For this review, take the finished solid that the model builds, in its own axes (mm). A direction names the side the tool comes from. Give positions to 0.01 mm unless a question says otherwise; leave off trailing zeros. Loops run counter-clockwise (first coordinate to the right, second up) from the corner with the lowest first, then second, coordinate; pieces in that order, holes last. Notation, with made-up numbers: (29, -34.75) - (39, -34.75) arc R8 cw to (39, -30.75) - close; hole circle Ø3 at (-9.75, 22.25). An arc over 180 degrees is marked (long way). Use CSV: the item, a comma, the result in double quotes. Start each with the question number.
1. Take a section at A-A on y = -35. Give the boundary of the cut face in (x, z), plus the area to 3 significant figures.
2. Take a section at D-D on y = 3.5. Give the boundary of the cut face in (x, z).
3. Mouldability with a two-part tool opening along Z and no side actions: class faces 1 (the flat face through (0, -70, -5)), 2 (the cylindrical face through (0.042, 57.196, 151.917)), 3 (the flat face through (0, -15, 65)), 4 (the cylindrical face through (0.042, 73.196, 151.917)) as pulls with the +Z half, pulls with the -Z half, needs draft (parallel to the pull), parting line crosses it, or undercut.
4. Take a section at C-C on x = 0.95. State how many separate pieces and enclosed holes the cut face has, plus the area to 3 significant figures.
5. For pin 1 (2 mm diameter, centred on x = 0, z = 82, fed in from -Y); pin 2 (12 mm diameter, centred on y = -16, z = 102.5, fed in from +X); pin 3 (1 mm diameter, centred on x = 1.5, y = -17, fed in from +Z), all flat-tipped, find the tip position at first contact; note any pin that passes through.
6. Wall thickness on line 1 (Y direction, x = 1, z = 55); line 2 (Y direction, x = -1, z = 50); line 3 (Y direction, x = 2.5, z = 152): over which ranges is each line inside the solid? List them lowest first.
7. For faces 5 (the cylindrical face through (0.04, -47.05, -6.54)), 6 (the flat face through (0.042, -63.695, 13.522)), list the 3-axis set-ups (+Z, -Z, +X, -X, +Y, -Y) from which the entire face can be reached by the end or side of a thin tool; tool diameter is ignored.
8. Take a section at B-B on y = 74. Give the boundary of the cut face in (x, z), plus the area to 3 significant figures.
```python
from build123d import *

# Parameters (mm, degrees)
SKETCH_1_R               = 6.025
EXTRUDE_1_DEPTH          = 3
SKETCH_2_R               = 3
SKETCH_2_R_2             = 2.1
CUT_EXTRUDE_1_DEPTH      = 10
SKETCH_4_R               = 2.1
CUT_EXTRUDE_3_DEPTH      = 10
CHAMFER_1_SIZE           = 10
FILLET_1_R               = 3
SKETCH_5_R               = 2.1
CUT_EXTRUDE_4_DEPTH      = 10
EXTRUDE_2_DEPTH          = 6
CUT_EXTRUDE_6_DEPTH      = 182.747077005
CUT_EXTRUDE_6_DEPTH_BACK = 182.747077005
EXTRUDE_START            = -6
SKETCH_7_R               = 2.1
EXTRUDE_3_DEPTH          = 6


with BuildPart() as part:
    # 草图1 → 凸台-拉伸1 (new, symmetric)
    with BuildSketch(Plane(origin=(0, 0, 0), x_dir=(0, 0, -1), z_dir=(1, 0, 0))):
        with BuildLine():
            Line((-60, -42.021540511), (0, -70))
            Line((0, -70), (12, -70))
            Line((12, -70), (12, 30))
            Line((12, 30), (-75.715728753, 30))
            Line((-75.715728753, 30), (-125.857864376, 80.142135624))
            ThreePointArc((-125.857864376, 80.142135624), (-154.142135624, 80.142135624), (-154.142135624, 51.857864376))
            Line((-154.142135624, 51.857864376), (-92.284271247, -10))
            Line((-92.284271247, -10), (-60, -10))
            Line((-60, -10), (-60, -42.021540511))
        make_face()
        Circle(SKETCH_1_R, mode=Mode.SUBTRACT)
    extrude(amount=EXTRUDE_1_DEPTH, both=True)

    # 草图2 → 切除-拉伸1 (cut)
    with BuildSketch(Plane(origin=(3, 0, 0), x_dir=(0, 0, -1), z_dir=(1, 0, 0))):
        with Locations((-140, 66)):
            Circle(SKETCH_2_R)
        with Locations((-140, 82)):
            Circle(SKETCH_2_R_2)
        with Locations((-126.143593539, 74)):
            Circle(SKETCH_2_R_2)
        with Locations((-126.143593539, 58)):
            Circle(SKETCH_2_R_2)
        with Locations((-140, 50)):
            Circle(SKETCH_2_R_2)
        with Locations((-153.856406461, 58)):
            Circle(SKETCH_2_R_2)
        with Locations((-153.856406461, 74)):
            Circle(SKETCH_2_R_2)
    extrude(amount=-CUT_EXTRUDE_1_DEPTH, mode=Mode.SUBTRACT)

    # 草图4 → 切除-拉伸3 (cut)
    with BuildSketch(Plane(origin=(3, 0, 0), x_dir=(0, 0, -1), z_dir=(1, 0, 0))):
        with Locations((-55, -15)):
            Circle(SKETCH_4_R)
        with Locations((-55, -35)):
            Circle(SKETCH_4_R)
        with Locations((7, -65)):
            Circle(SKETCH_4_R)
        with Locations((7, -45)):
            Circle(SKETCH_4_R)
        with Locations((-8, -60.75264914)):
            Circle(SKETCH_4_R)
        with Locations((-26.126155741, -52.300283905)):
            Circle(SKETCH_4_R)
        with Locations((-44.252311481, -43.84791867)):
            Circle(SKETCH_4_R)
    extrude(amount=-CUT_EXTRUDE_3_DEPTH, mode=Mode.SUBTRACT)

    # 倒角1
    chamfer_1_edges = [part.edges().sort_by_distance(p)[0] for p in [
        (0, -10, 60),
    ]]
    chamfer(chamfer_1_edges, length=CHAMFER_1_SIZE)

    # 圆角1
    fillet_1_edges = [part.edges().sort_by_distance(p)[0] for p in [
        (0, -20, 60),
        (0, -10, 70),
        (0, 30, -12),
        (0, -70, -12),
        (0, -70, 0),
        (0, -42.021540511, 60),
        (0, -10, 92.284271247),
        (0, 30, 75.715728753),
    ]]
    fillet(fillet_1_edges, radius=FILLET_1_R)

    # 草图5 → 切除-拉伸4 (cut)
    with BuildSketch(Plane(origin=(3, 0, 0), x_dir=(0, 0, -1), z_dir=(1, 0, 0))):
        with Locations((-110, 57.213203436)):
            Circle(SKETCH_5_R)
        with Locations((-88.786796564, 36)):
            Circle(SKETCH_5_R)
        with Locations((-109.946763354, 14.785654888)):
            Circle(SKETCH_5_R)
        with Locations((-131.214342006, 35.94434337)):
            Circle(SKETCH_5_R)
        with Locations((-58, 25)):
            Circle(SKETCH_5_R)
        with Locations((-28, 25)):
            Circle(SKETCH_5_R)
    extrude(amount=-CUT_EXTRUDE_4_DEPTH, mode=Mode.SUBTRACT)

    # 草图6 → 凸台-拉伸2 (add)
    with BuildSketch(Plane.ZY.offset(3)):
        with BuildLine():
            Line((36.127383127, -53.153524579), (26.084776747, -57.836468842))
            ThreePointArc((26.084776747, -57.836468842), (30.261373424, -57.503051447), (33.637803948, -59.983947227))
            ThreePointArc((33.637803948, -59.983947227), (46.226182617, -63.56307787), (51.576063312, -51.619199512))
            ThreePointArc((51.576063312, -51.619199512), (51.845914592, -47.438014603), (54.785991728, -44.452872497))
            Line((54.785991728, -44.452872497), (44.743385348, -49.13581676))
            ThreePointArc((44.743385348, -49.13581676), (47.139529245, -51.355820594), (48.025, -54.5))
            ThreePointArc((48.025, -54.5), (41.322464636, -60.486783012), (36.127383127, -53.153524579))
        make_face()
    extrude(amount=-EXTRUDE_2_DEPTH)

    # 草图6<3> → 切除-拉伸6 (cut, two sides: drawn at the far end of the back side and taken through both)
    with BuildSketch(Plane.ZY.offset(3).offset(-CUT_EXTRUDE_6_DEPTH_BACK)):
        with BuildLine():
            ThreePointArc((44.743385348, -49.13581676), (39.453724973, -49.039495583), (36.127383127, -53.153524579))
            Line((36.127383127, -53.153524579), (44.743385348, -49.13581676))
        make_face()
        with BuildLine():
            Line((44.743385348, -49.13581676), (36.127383127, -53.153524579))
            ThreePointArc((36.127383127, -53.153524579), (41.322464636, -60.486783012), (48.025, -54.5))
            ThreePointArc((48.025, -54.5), (47.139529245, -51.355820594), (44.743385348, -49.13581676))
        make_face()
    extrude(amount=CUT_EXTRUDE_6_DEPTH + CUT_EXTRUDE_6_DEPTH_BACK, mode=Mode.SUBTRACT)

    # 草图7 → 凸台-拉伸3 (add)
    with BuildSketch(Plane.ZY.offset(3).offset(EXTRUDE_START)):
        with BuildLine():
            ThreePointArc((98.29636037, 60.699261849), (101.887641952, 59.532632956), (101.49301897, 55.777290218))
            Line((101.49301897, 55.777290218), (125.857864376, 80.142135624))
            ThreePointArc((125.857864376, 80.142135624), (129.106517373, 82.772955502), (132.83107829, 84.671008583))
            Line((132.83107829, 84.671008583), (-10.075338256, 29.800651288))
            ThreePointArc((-10.075338256, 29.800651288), (-9.546830018, 29.949741841), (-9, 30))
            Line((-9, 30), (34.524823416, 30))
            ThreePointArc((34.524823416, 30), (31.575081575, 32.453169982), (33.44948516, 35.800651288))
            Line((33.44948516, 35.800651288), (98.29636037, 60.699261849))
        make_face()
        with Locations((44.499091861, 45.39915608)):
            Circle(SKETCH_7_R, mode=Mode.SUBTRACT)
        with Locations((63.170100444, 52.56807779)):
            Circle(SKETCH_7_R, mode=Mode.SUBTRACT)
        with Locations((81.841109028, 59.736999499)):
            Circle(SKETCH_7_R, mode=Mode.SUBTRACT)
    extrude(amount=EXTRUDE_3_DEPTH)


solid = part.part
```
Check result:
1,outline,"(-3, -12) - (3, -12) - (3, 52.9) - (-3, 52.9) - close; (-3, 57.1) - (3, 57.1) - (3, 60) - (-3, 60) - close"
1,area,"407 mm²"
2,outline,"(-3, -12) - (3, -12) - (3, -4.9) - (-3, -4.9) - close; (-3, 4.9) - (3, 4.9) - (3, 105.78) - (-3, 105.78) - close"
3,face 1,"needs draft"
3,face 2,"undercut"
3,face 3,"pulls with the +Z half"
3,face 4,"undercut"
4,separate pieces,"1"
4,enclosed holes,"26"
4,area,"12,200 mm²"
5,pin 1,"stops at y = -10"
5,pin 2,"passes through"
5,pin 3,"stops at z = 63.5"
6,line 1,"y = -44.35 to -37.1, -32.9 to -17.1, -12.9 to 30, 44.08 to 54.79"
6,line 2,"y = -60.5 to 30, 42.16 to 52.87"
6,line 3,"y = 49.72 to 57.02, 58.98 to 73.02, 74.98 to 82"
7,face 5,"+X, -X"
7,face 6,"+X, -X, -Y"
8,outline,"(-3, 105.04) - (3, 105.04) - (3, 124.04) - (-3, 124.04) - close; (-3, 128.24) - (3, 128.24) - (3, 151.76) - (-3, 151.76) - close; (-3, 155.96) - (3, 155.96) - (3, 158.33) - (-3, 158.33) - close"
8,area,"269 mm²"
